Read the model definition and answer for the solid it produces. Units are mm, in the model's axes. Face numbers are marked on the shaded views. A direction names the side the tool comes from. Give positions to 0.01 mm unless a question says otherwise; leave off trailing zeros. Loops run counter-clockwise (first coordinate to the right, second up) from the corner with the lowest first, then second, coordinate; pieces in that order, holes last.
(1) Straight lines are drawn through the part: probe 1 along Z at (x, y) = (0, -148); probe 2 along Z at (x, y) = (9.5, -15); probe 3 along X at (y, z) = (-175, 2.5). For each, find the intervals that lie inside material, in ascending order.
(2) Each of these flat-tipped pins is pushed along its axis until it touches: P1, Ø4, axis at x = 15, y = -132, coming from the +Z side; P2, Ø12.5, axis at y = -42.5, z = -19.5, coming from the +X side; P3, Ø4.5, axis at x = -19.5, y = -40.5, coming from the +Z side; P4, Ø5, axis at x = 10.5, y = -158, coming from the -Z side. Where does it stop, or does it pass through?
(3) Find section C-C, the plane z = 5. Write down the section's boundary in (x, y).
(4) Which of the six approach directions +Z, -Z, +X, -X, +Y, -Y give full straight-line access (tool end or side, diameter ignored) to the marked faces 1, 2, 3 and 4?
(5) Find section B-B, the plane y = -196. Write down the section's boundary in (x, z).
(6) Find section A-A, the plane z = -5.5. Write down the section's boundary in (x, y), then the cut area to 3 significant figures.
(7) Determine the mould class of the marked faces 5, 6, 7 and 8 for opening direction X: pulls with the +X half, pulls with the -X half, needs draft (parallel to the pull), parting line crosses it, or undercut.
```python
from build123d import *

# Parameters (mm, degrees)
F0_R     = 11.65
F0_R_2   = 11
F1_DEPTH = 220
F3_DEPTH = 0.8
F4_COUNT = 8


with BuildPart() as f1:
    # F0 (on Front) → F1 (new body)
    with BuildSketch(Plane.XZ):
        Circle(F0_R)
        Circle(F0_R_2, mode=Mode.SUBTRACT)
    extrude(amount=F1_DEPTH)

    # F2 (on Right) → F3 (join)
    with BuildSketch(Plane.YZ):
        Polygon((-67.270614, 11.36047), (0, 11.36047), (0, 20.928832), (-40.592879, 27.307741), (-31.023696, 18.319281), (-60.311206, 22.378588), align=None)
    extrude(amount=F3_DEPTH)

    # F4: F1 ×8 about axis
    f4_axis = Axis((0, 0, 0), (0, -1, 0))


with BuildPart() as f1_1:
    add(f1.part)
    for i in range(1, F4_COUNT):
        add(f1.part.rotate(f4_axis, i * 360 / F4_COUNT))


solid = f1_1.part
```
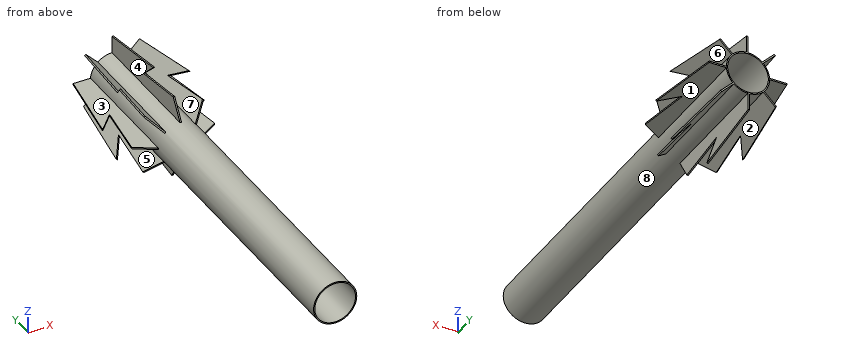
Entries:
1. probe 1: z = -11.65 to -11, 11 to 11.65
1. probe 2: z = -10.63 to -9.5, -6.74 to -5.55, 5.55 to 6.74, 8.37 to 9.5
1. probe 3: x = -11.38 to -10.71, 10.71 to 11.38
2. P1: passes through
2. P2: stops at x = 19.31
2. P3: stops at z = 19.88
2. P4: stops at z = -8.47
3. outline: (-10.52, -220) - (-9.8, -220) - (-9.8, 0) - (-10.52, 0) - close; (9.8, -220) - (10.52, -220) - (10.52, 0) - (9.8, 0) - close
4. face 1: +X, +Y, -Y
4. face 2: -Z, +Y, -Y
4. face 3: -X, +Y, -Y
4. face 4: +Z, +Y, -Y
5. outline: circle Ø23.3 at (0, 0); hole circle Ø22 at (0, 0)
6. outline: (-10.27, -220) - (-9.53, -220) - (-9.53, 0) - (-10.27, 0) - close; (9.53, -220) - (10.27, -220) - (10.27, 0) - (9.53, 0) - close
6. area: 327 mm2
7. face 5: pulls with the -X half
7. face 6: pulls with the +X half
7. face 7: undercut
7. face 8: undercut
